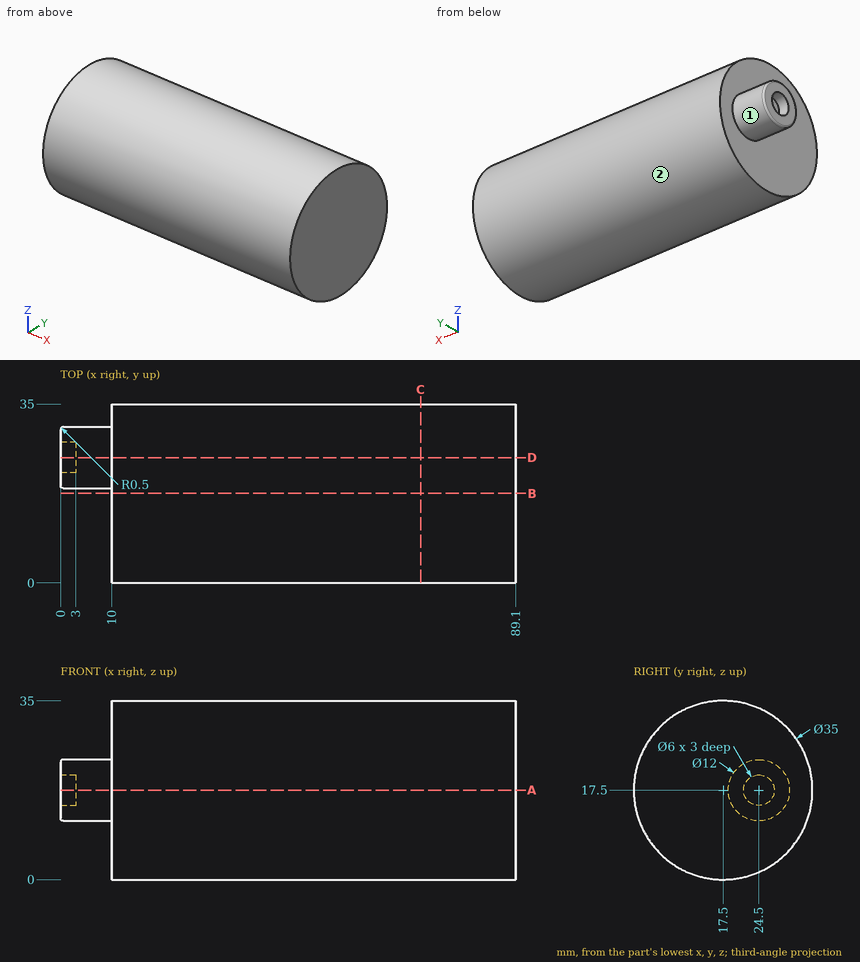
Study the drawing (mm; zero at the part's minimum x, y, z) and answer. A direction names the side the tool comes from. Round coordinates to 2 decimals unless told otherwise and drop trailing zeros. Loops run counter-clockwise (first coordinate to the right, second up) from the corner with the lowest first, then second, coordinate; pieces in that order, holes last.
Q1. Section C-C, the plane x = 70.5 is taken. Determine the outline of the cut face in (y, z).
Q2. Given pin 1 Ø8 at (x, y) = (45.5, 26) entering from -Z; pin 2 Ø12 at (x, y) = (41.5, 18.5) entering from -Z; pin 3 Ø4 at (x, z) = (79, 13.5) entering from +Y; pin 4 Ø2 at (y, z) = (18, 30) entering from -X, each flat-ended and moving along its own axis, determine where each tip first touches the part or whether it passes through.
Q3. Section B-B, the plane y = 17.5 is taken. Determine the outline of the cut face in (x, z), then the cut area to 3 significant figures.
Q4. Section D-D, the plane y = 24.5 is taken. Determine the outline of the cut face in (x, z).
Q5. Section A-A, the plane z = 17.5 is taken. Determine the outline of the cut face in (x, y).
Q6. Which of the six approach directions +Z, -Z, +X, -X, +Y, -Y give full straight-line access (tool end or side, diameter ignored) to the marked faces 1 and 2?
Q7. Find the intervals of material crossed by line 1 (Y direction, x = 1.9, z = 17.5); line 2 (X direction, y = 22, z = 10); line 3 (Z direction, x = 45.5, y = 17), in increasing order.
Completed:
1. outline: circle Ø35 at (17.5, 17.5)
2. pin 1: stops at z = 0.59
2. pin 2: stops at z = 0
2. pin 3: stops at y = 34.89
2. pin 4: stops at x = 10
3. outline: (10, 0) - (89.1, 0) - (89.1, 35) - (10, 35) - close
3. area: 2,770 mm2
4. outline: (0, 12) arc R0.5 ccw to (0.5, 11.5) - (10, 11.5) - (10, 1.46) - (89.1, 1.46) - (89.1, 33.54) - (10, 33.54) - (10, 23.5) - (0.5, 23.5) arc R0.5 ccw to (0, 23) - (0, 20.5) - (3, 20.5) - (3, 14.5) - (0, 14.5) - close
5. outline: (0, 19) arc R0.5 ccw to (0.5, 18.5) - (10, 18.5) - (10, 0) - (89.1, 0) - (89.1, 35) - (10, 35) - (10, 30.5) - (0.5, 30.5) arc R0.5 ccw to (0, 30) - (0, 27.5) - (3, 27.5) - (3, 21.5) - (0, 21.5) - close
6. face 1: -X
6. face 2: +X, -X
7. line 1: y = 18.5 to 21.5, 27.5 to 30.5
7. line 2: x = 10 to 89.1
7. line 3: z = 0.01 to 34.99
